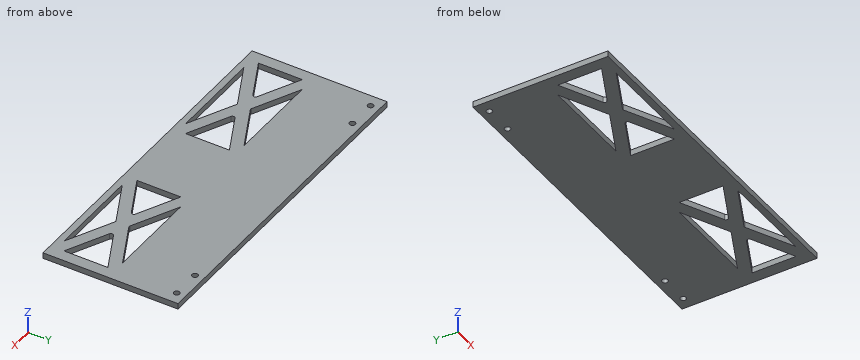
```python
from build123d import *

# Parameters (mm, degrees)
SKETCH6_W           = 286.5
SKETCH6_H           = 180
BOSS_EXTRUDE3_DEPTH = 5
SKETCH7_R           = 2.5
CUT_EXTRUDE1_DEPTH  = 13
SKETCH8_W           = 286.5
SKETCH8_H           = 64.5
CUT_EXTRUDE2_DEPTH  = 6


with BuildPart() as part:
    # Sketch6 → Boss-Extrude3 (new body)
    with BuildSketch(Plane.XY):
        with Locations((0, 90)):
            Rectangle(SKETCH6_W, SKETCH6_H)
    extrude(amount=BOSS_EXTRUDE3_DEPTH)

    # Sketch7 → Cut-Extrude1 (cut)
    with BuildSketch(Plane.XY.offset(5)):
        with Locations((-132.85, 172.5)):
            Circle(SKETCH7_R)
        with Locations((-107.85, 172.5)):
            Circle(SKETCH7_R)
        with BuildLine():
            Line((-82.374047462, 100.988572935), (-43.351346631, 120))
            Line((-43.351346631, 120), (-123.148653369, 120))
            Line((-123.148653369, 120), (-84.125952538, 100.988572935))
            ThreePointArc((-84.125952538, 100.988572935), (-83.25, 100.786546002), (-82.374047462, 100.988572935))
        make_face()
        with BuildLine():
            Line((-133.25, 113.797626904), (-133.25, 76.202373096))
            Line((-133.25, 76.202373096), (-98.356648563, 93.202026933))
            ThreePointArc((-98.356648563, 93.202026933), (-97.232601102, 95), (-98.356648563, 96.797973067))
            Line((-98.356648563, 96.797973067), (-133.25, 113.797626904))
        make_face()
        with BuildLine():
            Line((-68.143351437, 93.202026933), (-33.25, 76.202373096))
            Line((-33.25, 76.202373096), (-33.25, 113.797626904))
            Line((-33.25, 113.797626904), (-68.143351437, 96.797973067))
            ThreePointArc((-68.143351437, 96.797973067), (-69.267398898, 95), (-68.143351437, 93.202026933))
        make_face()
        with BuildLine():
            Line((-43.351346631, 70), (-82.374047462, 89.011427065))
            ThreePointArc((-82.374047462, 89.011427065), (-83.25, 89.213453998), (-84.125952538, 89.011427065))
            Line((-84.125952538, 89.011427065), (-123.148653369, 70))
            Line((-123.148653369, 70), (-43.351346631, 70))
        make_face()
        with BuildLine():
            Line((-43.351346631, 60), (-123.148653369, 60))
            Line((-123.148653369, 60), (-84.125952538, 40.988572935))
            ThreePointArc((-84.125952538, 40.988572935), (-83.25, 40.786546002), (-82.374047462, 40.988572935))
            Line((-82.374047462, 40.988572935), (-43.351346631, 60))
        make_face()
        with BuildLine():
            Line((-98.356648563, 36.797973067), (-133.25, 53.797626904))
            Line((-133.25, 53.797626904), (-133.25, 16.202373096))
            Line((-133.25, 16.202373096), (-98.356648563, 33.202026933))
            ThreePointArc((-98.356648563, 33.202026933), (-97.232601102, 35), (-98.356648563, 36.797973067))
        make_face()
        with BuildLine():
            Line((-33.25, 16.202373096), (-33.25, 53.797626904))
            Line((-33.25, 53.797626904), (-68.143351437, 36.797973067))
            ThreePointArc((-68.143351437, 36.797973067), (-69.267398898, 35), (-68.143351437, 33.202026933))
            Line((-68.143351437, 33.202026933), (-33.25, 16.202373096))
        make_face()
        with BuildLine():
            Line((-84.125952538, 29.011427065), (-123.148653369, 10))
            Line((-123.148653369, 10), (-43.351346631, 10))
            Line((-43.351346631, 10), (-82.374047462, 29.011427065))
            ThreePointArc((-82.374047462, 29.011427065), (-83.25, 29.213453998), (-84.125952538, 29.011427065))
        make_face()
        with BuildLine():
            Line((84.125952538, 100.988572935), (123.148653369, 120))
            Line((123.148653369, 120), (43.351346631, 120))
            Line((43.351346631, 120), (82.374047462, 100.988572935))
            ThreePointArc((82.374047462, 100.988572935), (83.25, 100.786546002), (84.125952538, 100.988572935))
        make_face()
        with BuildLine():
            Line((33.25, 113.797626904), (33.25, 76.202373096))
            Line((33.25, 76.202373096), (68.143351437, 93.202026933))
            ThreePointArc((68.143351437, 93.202026933), (69.267398898, 95), (68.143351437, 96.797973067))
            Line((68.143351437, 96.797973067), (33.25, 113.797626904))
        make_face()
        with BuildLine():
            Line((98.356648563, 93.202026933), (133.25, 76.202373096))
            Line((133.25, 76.202373096), (133.25, 113.797626904))
            Line((133.25, 113.797626904), (98.356648563, 96.797973067))
            ThreePointArc((98.356648563, 96.797973067), (97.232601102, 95), (98.356648563, 93.202026933))
        make_face()
        with BuildLine():
            Line((43.351346631, 70), (123.148653369, 70))
            Line((123.148653369, 70), (84.125952538, 89.011427065))
            ThreePointArc((84.125952538, 89.011427065), (83.25, 89.213453998), (82.374047462, 89.011427065))
            Line((82.374047462, 89.011427065), (43.351346631, 70))
        make_face()
        with BuildLine():
            Line((43.351346631, 60), (82.374047462, 40.988572935))
            ThreePointArc((82.374047462, 40.988572935), (83.25, 40.786546002), (84.125952538, 40.988572935))
            Line((84.125952538, 40.988572935), (123.148653369, 60))
            Line((123.148653369, 60), (43.351346631, 60))
        make_face()
        with BuildLine():
            Line((68.143351437, 36.797973067), (33.25, 53.797626904))
            Line((33.25, 53.797626904), (33.25, 16.202373096))
            Line((33.25, 16.202373096), (68.143351437, 33.202026933))
            ThreePointArc((68.143351437, 33.202026933), (69.267398898, 35), (68.143351437, 36.797973067))
        make_face()
        with BuildLine():
            Line((133.25, 16.202373096), (133.25, 53.797626904))
            Line((133.25, 53.797626904), (98.356648563, 36.797973067))
            ThreePointArc((98.356648563, 36.797973067), (97.232601102, 35), (98.356648563, 33.202026933))
            Line((98.356648563, 33.202026933), (133.25, 16.202373096))
        make_face()
        with BuildLine():
            Line((82.374047462, 29.011427065), (43.351346631, 10))
            Line((43.351346631, 10), (123.148653369, 10))
            Line((123.148653369, 10), (84.125952538, 29.011427065))
            ThreePointArc((84.125952538, 29.011427065), (83.25, 29.213453998), (82.374047462, 29.011427065))
        make_face()
        with Locations((107.85, 172.5)):
            Circle(SKETCH7_R)
        with Locations((132.85, 172.5)):
            Circle(SKETCH7_R)
    extrude(amount=-CUT_EXTRUDE1_DEPTH, mode=Mode.SUBTRACT)

    # Sketch8 → Cut-Extrude2 (cut, through all)
    with BuildSketch(Plane.XY.offset(5)):
        with Locations((0, 32.25)):
            Rectangle(SKETCH8_W, SKETCH8_H)
    extrude(amount=-CUT_EXTRUDE2_DEPTH, mode=Mode.SUBTRACT)


solid = part.part
```
The model under review builds one solid part; all positions refer to its coordinate system, in mm. Round coordinates to 2 decimals unless told otherwise and drop trailing zeros. Order: outer loops, then holes, each group sorted by start corner. A loop starts at its lowest first (then second) coordinate and runs counter-clockwise, first axis right, second up.
Item 1: Add section A-A, the plane x = 107.85. State the section outline as (y, z) points, and give its area (3 significant figures).
Working result:
outline: (64.5, 0) - (70, 0) - (70, 5) - (64.5, 5) - close; (77.45, 0) - (88.58, 0) - (88.58, 5) - (77.45, 5) - close; (101.42, 0) - (112.55, 0) - (112.55, 5) - (101.42, 5) - close; (120, 0) - (170, 0) - (170, 5) - (120, 5) - close; (175, 0) - (180, 0) - (180, 5) - (175, 5) - close
area: 414 mm2
Item 2: Add section C-C, the plane z = 3.55. Count the separate pieces of the cut face and the enclosed holes in it, and give its area (3 significant figures).
Working result:
separate pieces: 1
enclosed holes: 12
area: 27,000 mm2
Item 3: Add section B-B, the plane x = -78. State the section outline as (y, z) points, and give its area (3 significant figures).
Working result:
outline: (64.5, 0) - (70, 0) - (70, 5) - (64.5, 5) - close; (86.88, 0) - (103.12, 0) - (103.12, 5) - (86.88, 5) - close; (120, 0) - (180, 0) - (180, 5) - (120, 5) - close
area: 409 mm2
Item 4: For pin 1 (8 mm diameter, centred on x = 132.85, y = 172.5, fed in from -Z), flat-tipped, find the tip position at first contact; note if it passes through.
Working result:
pin 1: stops at z = 0
Item 5: To check wall thickness, follow probe 1 along X at (y, z) = (172.5, 1.95); probe 2 along Y at (x, z) = (-132.85, 2.45); probe 3 along Y at (x, z) = (89.5, 2.4). State the ranges of each line that lie inside material, in increasing order.
Working result:
probe 1: x = -143.25 to -135.35, -130.35 to -110.35, -105.35 to 105.35, 110.35 to 130.35, 135.35 to 143.25
probe 2: y = 64.5 to 76.4, 113.6 to 170, 175 to 180
probe 3: y = 64.5 to 70, 86.39 to 103.61, 120 to 180
